Verification items for the finished model (mm, model axes). Face numbers are marked on the shaded views. A direction names the side the tool comes from. Coordinates: 2 decimals unless noted, no trailing zeros. Loops run counter-clockwise (first coordinate to the right, second up) from the corner with the lowest first, then second, coordinate; pieces in that order, holes last.
Q1. Material ranges on probe 1 along Z at (x, y) = (11.5, -6.5); probe 2 along X at (y, z) = (3, 27.5); probe 3 along Y at (x, z) = (-4.5, 24.5), recorded low to high.
Q2. Sectioned sample at A-A (x = 0). Enter the section's corners in (y, z).
Q3. Access from +Z, -Z, +X, -X, +Y, -Y to the whole of each face (thin tool, end or side, straight path). Record for the marked faces 1 and 2.
Q4. Go/stop test with flat-tipped pins: P1, Ø3, axis at x = -7.5, z = 8.5, coming from the -Y side; P2, Ø4, axis at x = -8, z = 25.5, coming from the +Y side; P3, Ø2, axis at y = 14, z = 4, coming from the -X side; P4, Ø6, axis at x = 8.5, z = 10.5, coming from the +Y side. Record where each tip stops, or that it passes through.
Q5. Sectioned sample at C-C (z = 25). Enter the section's corners in (x, y).
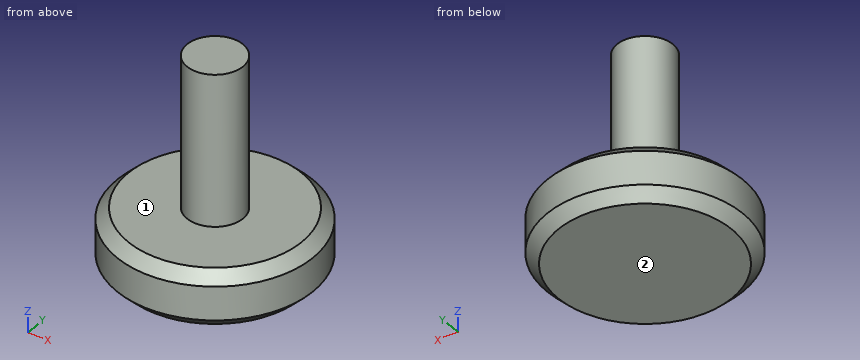
```python
from build123d import *

# Parameters (mm, degrees)
F0_R     = 17.5
F1_DEPTH = 10
F2_R     = 5
F3_DEPTH = 27
F4_SIZE  = 2


with BuildPart() as f1:
    # F0 (on Top) → F1 (new body)
    with BuildSketch(Plane.XY):
        Circle(F0_R)
    extrude(amount=F1_DEPTH)

    # F2 (on face) → F3 (join)
    with BuildSketch(Plane.XY.offset(10)):
        Circle(F2_R)
    extrude(amount=F3_DEPTH)

    # F4
    f4_edges = [f1.edges().sort_by_distance(p)[0] for p in [
        (-17.5, 0, 10),
        (-17.5, 0, 0),
    ]]
    chamfer(f4_edges, length=F4_SIZE)


solid = f1.part
```
Geometry check:
1. probe 1: z = 0 to 10
1. probe 2: x = -4 to 4
1. probe 3: y = -2.18 to 2.18
2. outline: (-17.5, 2) - (-15.5, 0) - (15.5, 0) - (17.5, 2) - (17.5, 8) - (15.5, 10) - (5, 10) - (5, 37) - (-5, 37) - (-5, 10) - (-15.5, 10) - (-17.5, 8) - close
3. face 1: +Z
3. face 2: -Z, +X, -X, +Y, -Y
4. P1: stops at y = -16.41
4. P2: passes through
4. P3: stops at x = -11.72
4. P4: stops at y = 16.11
5. outline: circle Ø10 at (0, 0)
